from build123d import *

# Parameters (mm, degrees)
SKETCH1_R           = 4
SKETCH1_W           = 42
SKETCH1_H           = 14
SKETCH1_W_2         = 40
BOSS_EXTRUDE1_DEPTH = 10
FILLET1_R           = 7
FILLET2_R           = 3


with BuildPart() as part:
    # Sketch1 → Boss-Extrude1 (new body)
    with BuildSketch(Plane(origin=(0, 0, 0), x_dir=(1, 0, 0), z_dir=(0, 1, 0))):
        with BuildLine():
            Line((-200, 12), (0, 12))
            ThreePointArc((0, 12), (12, 0), (0, -12))
            Line((0, -12), (-200, -12))
            ThreePointArc((-200, -12), (-205.477225575, -10.677078252), (-209.746794345, -7))
            Line((-209.746794345, -7), (-229.746794345, -7))
            Line((-229.746794345, -7), (-229.746794345, 7))
            Line((-229.746794345, 7), (-209.746794345, 7))
            ThreePointArc((-209.746794345, 7), (-205.477225575, 10.677078252), (-200, 12))
        make_face()
        with Locations(Location((-200, 0, 0), (0, 0, 270))):
            Circle(SKETCH1_R, mode=Mode.SUBTRACT)
        with Locations(Location((0, 0, 0), (0, 0, 270))):
            Circle(SKETCH1_R, mode=Mode.SUBTRACT)
        with Locations((-167, 0)):
            Rectangle(SKETCH1_W, SKETCH1_H, mode=Mode.SUBTRACT)
        with Locations((-122, 0)):
            Rectangle(SKETCH1_W_2, SKETCH1_H, mode=Mode.SUBTRACT)
        with Locations((-78, 0)):
            Rectangle(SKETCH1_W_2, SKETCH1_H, mode=Mode.SUBTRACT)
        with Locations((-33, 0)):
            Rectangle(SKETCH1_W, SKETCH1_H, mode=Mode.SUBTRACT)
    extrude(amount=BOSS_EXTRUDE1_DEPTH)

    # Fillet1
    fillet1_edges = [part.edges().sort_by_distance(p)[0] for p in [
        (-142, 5, -7),
        (-98, 5, -7),
        (-54, 5, -7),
        (-58, 5, -7),
        (-12, 5, -7),
        (-102, 5, -7),
        (-146, 5, -7),
        (-146, 5, 7),
        (-102, 5, 7),
        (-58, 5, 7),
        (-12, 5, 7),
        (-54, 5, 7),
        (-98, 5, 7),
        (-142, 5, 7),
        (-188, 5, 7),
        (-188, 5, -7),
        (-209.746794345, 5, 7),
        (-209.746794345, 5, -7),
    ]]
    fillet(fillet1_edges, radius=FILLET1_R - 0.0001)  # a hair under: the kernel refuses the full size

    # Fillet2
    fillet2_edges = [part.edges().sort_by_distance(p)[0] for p in [
        (-229.746794345, 5, 7),
        (-229.746794345, 5, -7),
    ]]
    fillet(fillet2_edges, radius=FILLET2_R)


solid = part.part
Model file for the job. Use its own axes, mm. A direction names the side the tool comes from. Give positions to 0.01 mm unless a question says otherwise; leave off trailing zeros. Loops run counter-clockwise (first coordinate to the right, second up) from the corner with the lowest first, then second, coordinate; pieces in that order, holes last. Notation, with made-up numbers: (21.5, -1.75) -> (44.5, -1.75) arc R15 cw to (44.5, 4.25) -> close; hole circle Ø9 at (-28, 26.25). An arc over 180 degrees is marked (long way). Use a Markdown table: item, result. Add a question column.
(1) Slice it at A-A on x = -161. List the corners of the cut face in (y, z).
(2) Wall check: line 1 along Z through (x, y) = (-26, 8); line 2 along X through (y, z) = (8.5, -6); line 3 along Z through (x, y) = (-104, 2.5). Give the ranges that are in metal, low to high.
(3) Mould opens along X. For faces 4 (the cylindrical face through (12, 5, 0)), 5 (the flat face through (-99, 5, 12)), 6 (the flat face through (-78, 5, -7)) say: +X half, -X half, draft (parallel to the pull), parting line (faces both ways), or undercut.
(4) Slice it at C-C on y = 5. Give the number of separate pieces and of enclosed holes in the cut face, and give its area (3 significant figures).
(5) Tool access for faces 1 (the flat face through (-220, 5, -7)), 2 (the flat face through (-107, 0, -8)), 3 (the flat face through (-122, 5, 7)): list every direction of +Z, -Z, +X, -X, +Y, -Y with a clear straight run to the whole face (end or side of a thin tool).
(6) Drop flat-ended pins along their axis: pin 1 Ø6 at (y, z) = (8.5, -4.5) entering from +X; pin 2 Ø6 at (x, y) = (-201, 2.5) entering from -Z. Give the stop position or say it passes through.
(7) Slice it at B-B on z = 2. List the corners of the cut face in (x, y).
Filled sheet:
| question | item | result |
|---|---|---|
| 1 | outline | (0, -12) -> (10, -12) -> (10, -7) -> (0, -7) -> close; (0, 7) -> (10, 7) -> (10, 12) -> (0, 12) -> close |
| 2 | line 1 | -12 to -7, 7 to 12 |
| 2 | line 2 | -228.98 to -184.61, -149.39 to -138.61, -105.39 to -94.61, -61.39 to -50.61, -15.39 to 10.39 |
| 2 | line 3 | -12 to -4.9, 4.9 to 12 |
| 3 | face 4 | +X half |
| 3 | face 5 | draft |
| 3 | face 6 | undercut |
| 4 | separate pieces | 1 |
| 4 | enclosed holes | 6 |
| 4 | area | 3,280 mm2 |
| 5 | face 1 | -Z, -X, +Y, -Y |
| 5 | face 2 | +Z, -Z, +X, -X, -Y |
| 5 | face 3 | +Y, -Y |
| 6 | pin 1 | x = 11.91 |
| 6 | pin 2 | z = -12 |
| 7 | outline | (-229.75, 0) -> (-203.46, 0) -> (-203.46, 10) -> (-229.75, 10) -> close; (-196.54, 0) -> (-187.71, 0) -> (-187.71, 10) -> (-196.54, 10) -> close; (-146.29, 0) -> (-141.71, 0) -> (-141.71, 10) -> (-146.29, 10) -> close; (-102.29, 0) -> (-97.71, 0) -> (-97.71, 10) -> (-102.29, 10) -> close; (-58.29, 0) -> (-53.71, 0) -> (-53.71, 10) -> (-58.29, 10) -> close; (-12.29, 0) -> (-3.46, 0) -> (-3.46, 10) -> (-12.29, 10) -> close; (3.46, 0) -> (11.83, 0) -> (11.83, 10) -> (3.46, 10) -> close |
